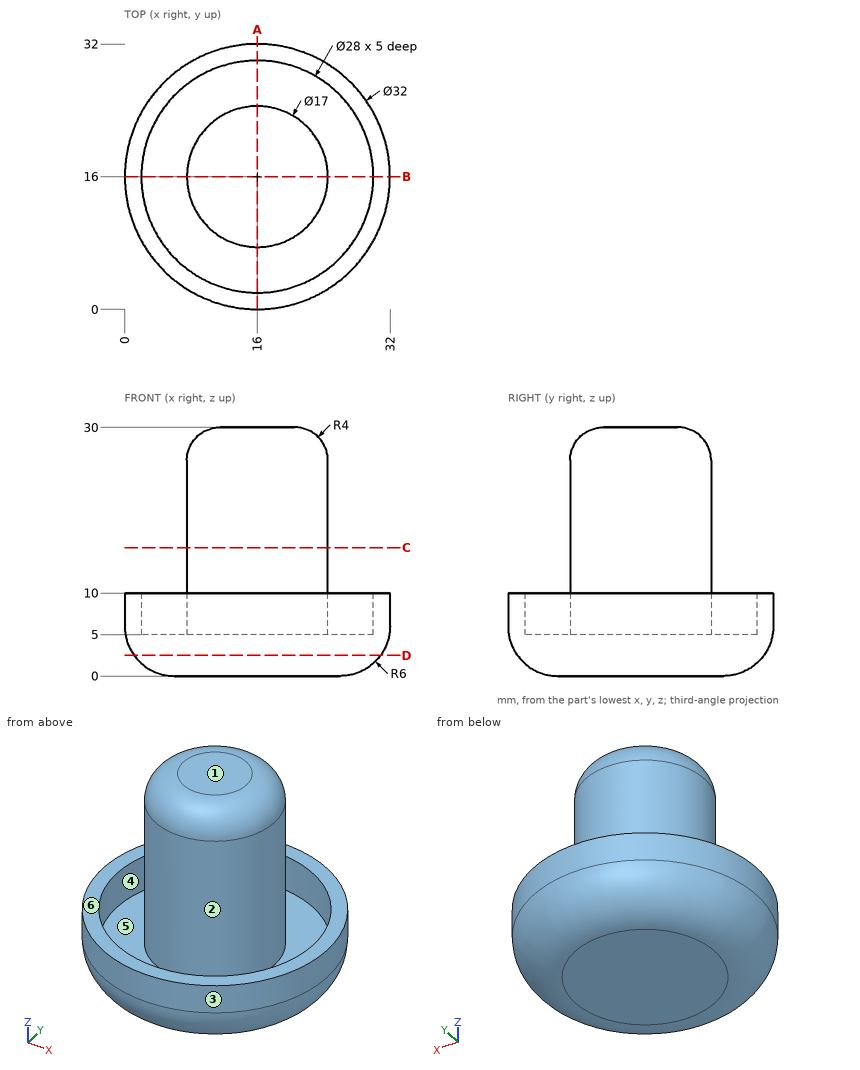
Job drawing, mm, ordinate dimensions from the low corner. One solid piece. A direction names the side the tool comes from. Give positions to 0.01 mm unless a question says otherwise; leave off trailing zeros. Order: outer loops, then holes, each group sorted by start corner. A loop starts at its lowest first (then second) coordinate and runs counter-clockwise, first axis right, second up. Notation, with made-up numbers: (-20, -38.75) - (17, -38.75) arc R11 ccw to (17, -17.75) - close; hole circle Ø8 at (66.25, -26). An arc over 180 degrees is marked (long way). One line per question, with ' | ' between items.
1. Drill centre lines: probe 1 along Y at (x, z) = (16, 7.7); probe 2 along Y at (x, z) = (5, 8.5); probe 3 along Z at (x, y) = (9, 11). Where is each one in solid material? Low to high.
Filled in:
probe 1: 0 to 2, 7.5 to 24.5, 30 to 32 | probe 2: 4.38 to 7.34, 24.66 to 27.62 | probe 3: 0 to 5
2. Pull direction Y, two halves, no side cores. Call the marked faces 3, 4, 5 and 6: +Y half, -Y half, draft (parallel to the pull), parting line (faces both ways), or undercut.
Filled in:
face 3: parting line | face 4: undercut | face 5: undercut | face 6: draft
3. Band-saw the part on C-C on z = 15.5. List the corners of the cut face in (x, y), then the cut area to 3 significant figures.
Filled in:
outline: circle Ø17 at (16, 16) | area: 227 mm²
4. Band-saw the part on A-A on x = 16. List the corners of the cut face in (y, z).
Filled in:
outline: (0, 6) arc R6 ccw to (6, 0) - (26, 0) arc R6 ccw to (32, 6) - (32, 10) - (30, 10) - (30, 5) - (24.5, 5) - (24.5, 26) arc R4 ccw to (20.5, 30) - (11.5, 30) arc R4 ccw to (7.5, 26) - (7.5, 5) - (2, 5) - (2, 10) - (0, 10) - close
5. Which spindle directions (+Z, -Z, +X, -X, +Y, -Y) get a long thin tool onto all of the face, cutting with end or side? Do the marked faces 1 and 2. Say none if no direction does.
Filled in:
face 1: +Z, +X, -X, +Y, -Y | face 2: +Z
6. Band-saw the part on D-D on z = 2.5. List the corners of the cut face in (x, y).
Filled in:
outline: circle Ø29.75 at (16, 16)
7. Drop flat-ended pins along their axis: P1, Ø5, axis at x = 15.5, y = 28, coming from the +Z side; P2, Ø1.5, axis at x = 23.5, y = 15.5, coming from the -Z side; P3, Ø3, axis at x = 26.5, z = 12.5, coming from the -Y side; P4, Ø4, axis at x = 16, y = 25, coming from the +Z side. Give the stop position or say it passes through.
Filled in:
P1: z = 10 | P2: z = 0 | P3: through | P4: z = 29.12
